Drawing for the job (mm, zero at the part's lowest x, y, z). A direction names the side the tool comes from. Round coordinates to 2 decimals unless told otherwise and drop trailing zeros. Write each loop counter-clockwise with the first axis right and the second up, starting at its lowest first coordinate (ties: lowest second). Pieces come first, ordered by that corner, then holes.
Item 1: Band-saw the part on B-B, the plane x = 10.5. Write the cut outline in (y, z).
Item 2: Wall check: probe 1 along Z at (x, y) = (7, 2); probe 2 along X at (y, z) = (5.5, 36); probe 3 along X at (y, z) = (4.75, 45.5). Give the ranges that are in metal, low to high.
Item 3: 3-axis set-ups, long thin cutter, end or side, ignore diameter. For the marked faces 4, 5, 6 and 7: which of +Z, -Z, +X, -X, +Y, -Y reach the whole face in a straight line?
Item 4: Band-saw the part on C-C, the plane z = 19.5. Write the cut outline in (x, y), then the cut area to 3 significant figures.
Item 5: Drop flat-ended pins along their axis: pin 1 Ø3 at (x, y) = (30, 2) entering from +Z; pin 2 Ø1.5 at (x, y) = (34, 3.5) entering from -Z; pin 3 Ø3.5 at (y, z) = (4.5, 54.5) entering from +X. Give the stop position or say it passes through.
Item 6: Band-saw the part on D-D, the plane x = 24. Write the cut outline in (y, z), then the cut area to 3 significant figures.
Item 7: Band-saw the part on A-A, the plane z = 44.5. Write the cut outline in (x, y), then the cut area to 3 significant figures.
Item 8: Mould opens along Z. For the marked faces 1, 2 and 3 say: +Z half, -Z half, draft (parallel to the pull), parting line (faces both ways), or undercut.
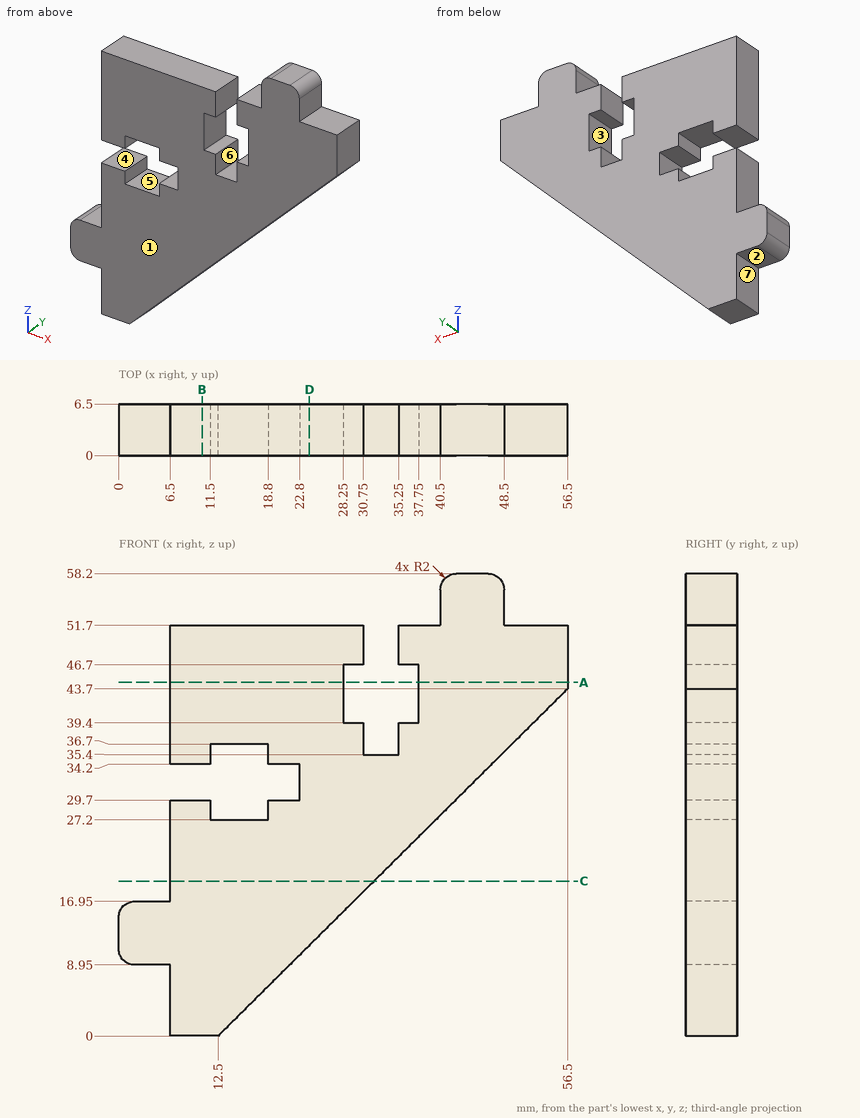
Results:
1. outline: (0, 0) - (6.5, 0) - (6.5, 29.7) - (0, 29.7) - close; (0, 34.2) - (6.5, 34.2) - (6.5, 51.7) - (0, 51.7) - close
2. probe 1: z = 0 to 29.7, 34.2 to 51.7
2. probe 2: x = 6.5 to 11.5, 18.8 to 30.75, 35.25 to 48.75
2. probe 3: x = 6.5 to 28.25, 37.75 to 56.5
3. face 4: -X, +Y, -Y
3. face 5: +Y, -Y
3. face 6: +Z, +Y, -Y
3. face 7: -Z, -X, +Y, -Y
4. outline: (6.5, 0) - (32.13, 0) - (32.13, 6.5) - (6.5, 6.5) - close
4. area: 167 mm2
5. pin 1: stops at z = 51.7
5. pin 2: stops at z = 20.61
5. pin 3: stops at x = 48.5
6. outline: (0, 11.42) - (6.5, 11.42) - (6.5, 51.7) - (0, 51.7) - close
6. area: 262 mm2
7. outline: (6.5, 0) - (28.25, 0) - (28.25, 6.5) - (6.5, 6.5) - close; (37.75, 0) - (56.5, 0) - (56.5, 6.5) - (37.75, 6.5) - close
7. area: 263 mm2
8. face 1: draft
8. face 2: -Z half
8. face 3: undercut
